Print and shaded views of the part. All mm, measured from the part's lowest x, y and z. Give positions to 0.01 mm unless a question says otherwise; leave off trailing zeros. Order: outer loops, then holes, each group sorted by start corner. A loop starts at its lowest first (then second) coordinate and runs counter-clockwise, first axis right, second up. Notation, with made-up numbers: (20, -10.5) - (72, -10.5) arc R21 cw to (72, 0.5) - close; hole circle Ø9 at (59, 65.5). An arc over 180 degrees is marked (long way). Answer in a Markdown table with one row per item.
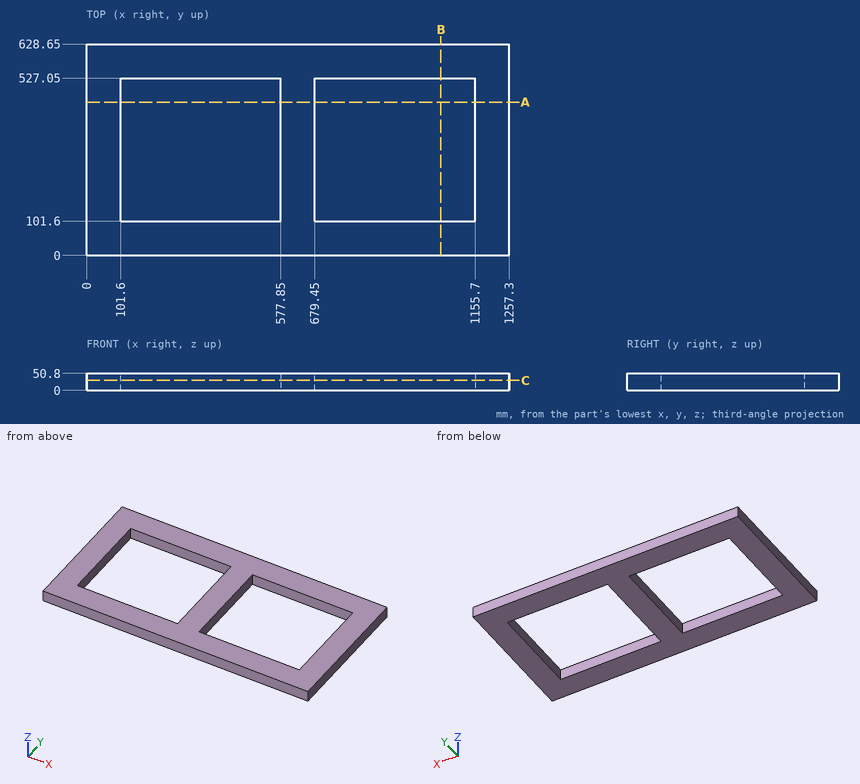
1. Probe line 1 (X direction, y = 389, z = 33); line 2 (Y direction, x = 1136, z = 14). List the from-to ranges inside material, lowest first.
Check result:
| item | result |
|---|---|
| line 1 | x = 0 to 101.6, 577.85 to 679.45, 1155.7 to 1257.3 |
| line 2 | y = 0 to 101.6, 527.05 to 628.65 |
2. Cut at A-A on y = 456. Write the cut outline in (x, z).
Check result:
| item | result |
|---|---|
| outline | (0, 0) - (101.6, 0) - (101.6, 50.8) - (0, 50.8) - close; (577.85, 0) - (679.45, 0) - (679.45, 50.8) - (577.85, 50.8) - close; (1155.7, 0) - (1257.3, 0) - (1257.3, 50.8) - (1155.7, 50.8) - close |
3. Cut at B-B on x = 1054. Write the cut outline in (y, z).
Check result:
| item | result |
|---|---|
| outline | (0, 0) - (101.6, 0) - (101.6, 50.8) - (0, 50.8) - close; (527.05, 0) - (628.65, 0) - (628.65, 50.8) - (527.05, 50.8) - close |
4. Cut at C-C on z = 30. Write the cut outline in (x, y), and give its area (3 significant figures).
Check result:
| item | result |
|---|---|
| outline | (0, 0) - (1257.3, 0) - (1257.3, 628.65) - (0, 628.65) - close; hole (101.6, 101.6) - (577.85, 101.6) - (577.85, 527.05) - (101.6, 527.05) - close; hole (679.45, 101.6) - (1155.7, 101.6) - (1155.7, 527.05) - (679.45, 527.05) - close |
| area | 385,000 mm² |
